Read the model definition and answer for the solid it produces. Units are mm, in the model's axes. A direction names the side the tool comes from. Coordinates: 2 decimals unless noted, no trailing zeros. Loops run counter-clockwise (first coordinate to the right, second up) from the corner with the lowest first, then second, coordinate; pieces in that order, holes last. Notation, with made-up numbers: M 38,41.5 L 95,41.5 A9 ccw 95,50.5 Z; hole C 27,43.25 d9. An arc over 180 degrees is marked long. Put each result on its own line as item: value.
from build123d import *

# Parameters (mm, degrees)
F0_W     = 116.999064
F0_H     = 113.067575
F1_DEPTH = 65.278
F2_R     = 12.7
F3_T     = -2.54
F4_R     = 24.811163
F5_DEPTH = 64.008
F6_SIZE  = 1.27


with BuildPart() as f1:
    # F0 (on Front) → F1 (new body)
    with BuildSketch(Plane.XZ):
        with Locations((-1.865206, -0.708006)):
            Rectangle(F0_W, F0_H)
    extrude(amount=F1_DEPTH)

    # F2
    f2_edges = [f1.edges().sort_by_distance(p)[0] for p in [
        (-1.865206, 0, 55.825781),
        (56.634326, -32.639, 55.825781),
        (56.634326, 0, -0.708006),
        (56.634326, -32.639, -57.241794),
        (-1.865206, 0, -57.241794),
        (-60.364738, -32.639, -57.241794),
        (-60.364738, 0, -0.708006),
        (-60.364738, -32.639, 55.825781),
    ]]
    fillet(f2_edges, radius=F2_R)

    # F3
    f3_openings = [f1.faces().sort_by_distance(p)[0] for p in [
        (-1.865206, -65.278, -0.708006),
    ]]
    offset(amount=F3_T, openings=f3_openings)

    # F4 (on face) → F5 (cut)
    with BuildSketch(Plane.XZ.offset(2.54)):
        Circle(F4_R)
    extrude(amount=-F5_DEPTH, mode=Mode.SUBTRACT)

    # F6
    f6_edges = [f1.edges().sort_by_distance(p)[0] for p in [
        (-1.865206, -65.278, 55.825781),
    ]]
    chamfer(f6_edges, length=F6_SIZE)


solid = f1.part
1) Find section D-D, the plane x = 42. Write down the section's boundary in (y, z).
Answer list:
outline: M -65.28,-55.97 L -64.01,-57.24 L -12.7,-57.24 A12.7 ccw 0,-44.54 L 0,43.13 A12.7 ccw -12.7,55.83 L -64.01,55.83 L -65.28,54.56 L -65.28,53.29 L -12.7,53.29 A10.16 cw -2.54,43.13 L -2.54,-44.54 A10.16 cw -12.7,-54.7 L -65.28,-54.7 Z
2) Which of the six approach directions +Z, -Z, +X, -X, +Y, -Y give full straight-line access (tool end or side, diameter ignored) to faces 1 (the cylindrical face through (51.039, -39.357, -51.805)), 2 (the conical face through (52.08, -65.06, 51.45))?
Answer list:
face 1: -Y
face 2: +Z, +X, -Y
3) Straight lines are drawn through the part: line 1 (Z direction, x = -5, y = -43.5); line 2 (X direction, y = -32.5, z = 41.5); line 3 (Y direction, x = -23, z = -25). For each, find the intervals that lie inside material, in ascending order. Write a range as [from, to].
Answer list:
line 1: z = [-57.24, -54.7], [53.29, 55.83]
line 2: x = [-60.36, -57.82], [54.09, 56.63]
line 3: y = [-2.54, 0]
4) Determine the mould class of faces 3 (the cylindrical face through (53.013, -3.819, -0.094)), 4 (the cylindrical face through (-1.224, -5.595, 50.389)), 5 (the conical face through (-55.81, -65.06, -52.87)) for opening direction Z: released by +Z, released by -Z, zero draft, split by the parting line, or undercut.
Answer list:
face 3: zero draft
face 4: undercut
face 5: released by -Z
5) Find section C-C, the plane z = 0. Write down the section's boundary in (x, y), plus the area to 3 significant figures.
Answer list:
outline: M -60.36,-64.01 L -59.09,-65.28 L -57.82,-65.28 L -57.82,-12.7 A10.16 cw -47.66,-2.54 L -24.81,-2.54 L -24.81,0 L -47.66,0 A12.7 ccw -60.36,-12.7 Z; M 24.81,-2.54 L 43.93,-2.54 A10.16 cw 54.09,-12.7 L 54.09,-65.28 L 55.36,-65.28 L 56.63,-64.01 L 56.63,-12.7 A12.7 ccw 43.93,0 L 24.81,0 Z
area: 463 mm^2
6) Given pin 1 Ø1 at (x, z) = (22, -33) entering from -Y, flat-ended and moving along its own axis, determine where the tip first touches the part or whether it passes through.
Answer list:
pin 1: stops at y = -2.54
7) Find section B-B, the plane y = -34. Write down the section's boundary in (x, z), plus the area to 3 significant figures.
Answer list:
outline: M -60.36,-44.54 A12.7 ccw -47.66,-57.24 L 43.93,-57.24 A12.7 ccw 56.63,-44.54 L 56.63,43.13 A12.7 ccw 43.93,55.83 L -47.66,55.83 A12.7 ccw -60.36,43.13 Z; hole M -57.82,-44.54 A10.16 ccw -47.66,-54.7 L 43.93,-54.7 A10.16 ccw 54.09,-44.54 L 54.09,43.13 A10.16 ccw 43.93,53.29 L -47.66,53.29 A10.16 ccw -57.82,43.13 Z
area: 1,090 mm^2
8) Find section A-A, the plane x = 0. Write down the section's boundary in (y, z), plus the area to 3 significant figures.
Answer list:
outline: M -65.28,-55.97 L -64.01,-57.24 L -12.7,-57.24 A12.7 ccw 0,-44.54 L 0,-24.81 L -2.54,-24.81 L -2.54,-44.54 A10.16 cw -12.7,-54.7 L -65.28,-54.7 Z; M -65.28,53.29 L -12.7,53.29 A10.16 cw -2.54,43.13 L -2.54,24.81 L 0,24.81 L 0,43.13 A12.7 ccw -12.7,55.83 L -64.01,55.83 L -65.28,54.56 Z
area: 453 mm^2
